Verification items for this drawing (mm, ordinates from the low corner). A direction names the side the tool comes from. Round coordinates to 2 decimals unless told otherwise and drop trailing zeros. Order: outer loops, then holes, each group sorted by start corner. A loop starts at its lowest first (then second) coordinate and runs counter-clockwise, first axis right, second up. Notation, with made-up numbers: M 26.25,29.5 L 84.25,29.5 A17 ccw 84.25,40.5 Z; hole C -24.5,-13 d2. An arc over 180 degrees is marked long. One line per item, written item: value. Start each with the question number.
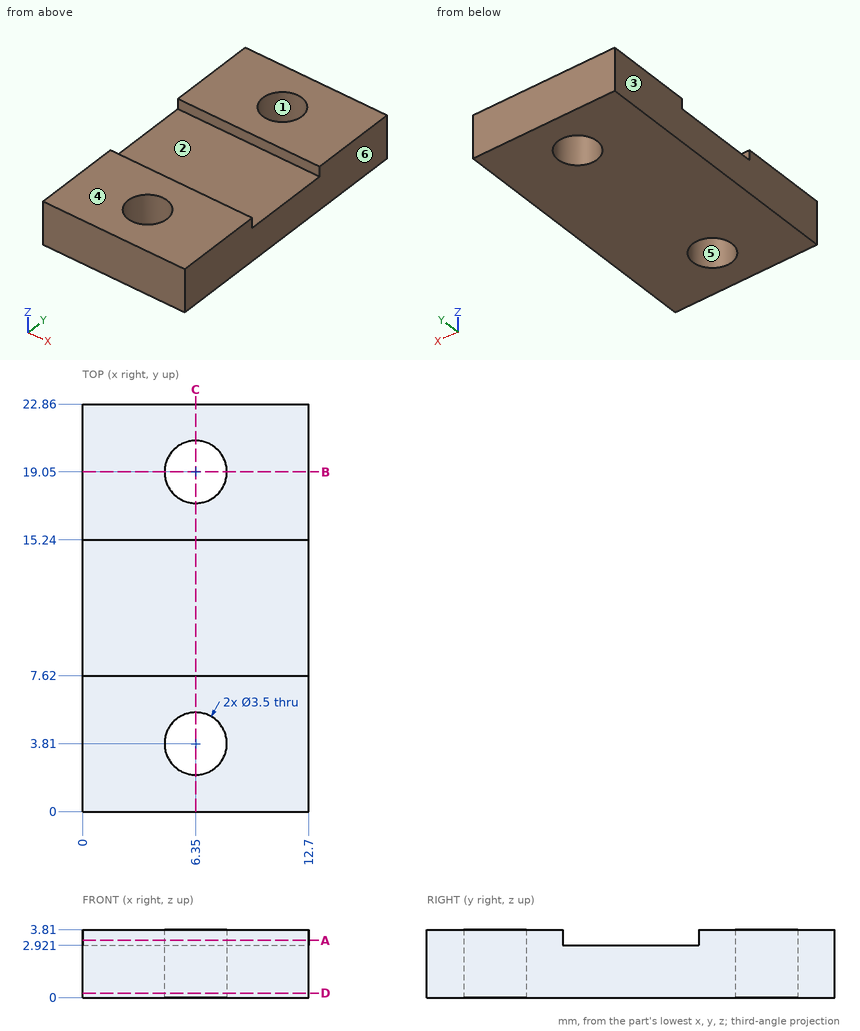
1. Section check A-A (z = 3.2). Record the cut outline in (x, y), and give its area (3 significant figures).
2. Section check D-D (z = 0.25). Record the cut outline in (x, y).
3. Scan lines: line 1 along Y through (x, z) = (6.35, 1); line 2 along Y through (x, z) = (6.35, 3); line 3 along Y through (x, z) = (4.5, 3.55). Record each from-to range of solid material in increasing order.
4. Section check C-C (x = 6.35). Record the cut outline in (y, z), and give its area (3 significant figures).
5. Section check B-B (y = 19.05). Record the cut outline in (x, z), and give its area (3 significant figures).
6. Draft check along X on the marked faces 3, 4, 5 and 6. Enter one of: released by +X, released by -X, zero draft, split by the parting line, or undercut.
7. Tool access check on the marked faces 1 and 2. Record the directions out of +Z, -Z, +X, -X, +Y, -Y that give a thin tool (end or side, any length) a straight path to the whole face; none if there is none.
8. Depth check by flat-ended pin: pin 1 (1 mm diameter, centred on x = 4, y = 14.5, fed in from +Z). Enter the tip coordinate at first touch or a pass-through.
Geometry check:
1. outline: M 0,0 L 12.7,0 L 12.7,7.62 L 0,7.62 Z; M 0,15.24 L 12.7,15.24 L 12.7,22.86 L 0,22.86 Z; hole C 6.35,3.81 d3.5; hole C 6.35,19.05 d3.5
1. area: 174 mm²
2. outline: M 0,0 L 12.7,0 L 12.7,22.86 L 0,22.86 Z; hole C 6.35,3.81 d3.5; hole C 6.35,19.05 d3.5
3. line 1: y = 0 to 2.06, 5.56 to 17.3, 20.8 to 22.86
3. line 2: y = 0 to 2.06, 5.56 to 7.62, 15.24 to 17.3, 20.8 to 22.86
3. line 3: y = 0 to 7.62, 15.24 to 22.86
4. outline: M 0,0 L 2.06,0 L 2.06,3.81 L 0,3.81 Z; M 5.56,0 L 17.3,0 L 17.3,3.81 L 15.24,3.81 L 15.24,2.92 L 7.62,2.92 L 7.62,3.81 L 5.56,3.81 Z; M 20.8,0 L 22.86,0 L 22.86,3.81 L 20.8,3.81 Z
4. area: 53.7 mm²
5. outline: M 0,0 L 4.6,0 L 4.6,3.81 L 0,3.81 Z; M 8.1,0 L 12.7,0 L 12.7,3.81 L 8.1,3.81 Z
5. area: 35.1 mm²
6. face 3: released by -X
6. face 4: zero draft
6. face 5: undercut
6. face 6: released by +X
7. face 1: +Z, -Z
7. face 2: +Z, +X, -X
8. pin 1: stops at z = 2.92
